The listing builds one solid part. Answer for the finished solid, in the listing's coordinates (mm). Face numbers are marked on the shaded views. A direction names the side the tool comes from. Round coordinates to 2 decimals unless told otherwise and drop trailing zeros. Write each loop counter-clockwise with the first axis right and the second up, starting at its lowest first coordinate (ties: lowest second). Pieces come first, ordered by that corner, then holes.
Item 1: A tool of negligible diameter and unlimited length cuts with its end or side. For the marked faces 4 and 5, from which of +Z, -Z, +X, -X, +Y, -Y can it reach the whole face along a straight path? Write none if from no direction.
Item 2: Find section D-D on y = 26.75. Give the vertices of the cut face in (x, z), then the cut area to 3 significant figures.
Item 3: Find the intervals of material crossed by probe 1 along Z at (x, y) = (0, 23.1); probe 2 along Y at (x, z) = (24.5, -21.5); probe 3 along Z at (x, y) = (2.5, 22.5), in increasing order.
Item 4: Each of these flat-tipped pins is pushed along its axis until it touches: pin 1 (6 mm diameter, centred on y = 25, z = 32, fed in from +X); pin 2 (2.5 mm diameter, centred on x = 0, z = -34.5, fed in from +Y); pin 3 (2.5 mm diameter, centred on x = 0, z = 32.5, fed in from -Y); pin 4 (2 mm diameter, centred on y = 22, z = -21, fed in from -X). Where does it stop, or does it pass through?
Item 5: Find section B-B on x = 17. Give the vertices of the cut face in (y, z), then the cut area to 3 significant figures.
Item 6: Find section A-A on z = -34.5. Give the vertices of the cut face in (x, y), then the cut area to 3 significant figures.
Item 7: Find section C-C on x = 0. Give the number of separate pieces and of enclosed holes in the cut face, then the cut area to 3 significant figures.
Item 8: For a pull along X with two mould halves and no side action, classify the marked faces 1, 2 and 3 as +X half, -X half, draft (parallel to the pull), parting line (faces both ways), or undercut.
Autodesk Inventor part; units mm, degrees
ref_plane "YZ Plane" through (0, 0, 0) normal (1, 0, 0) x (0, 1, 0)
ref_plane "XZ Plane" through (0, 0, 0) normal (0, 1, 0) x (-1, 0, 0)
ref_plane "XY Plane" through (0, 0, 0) normal (0, 0, 1) x (1, 0, 0)
sketch "スケッチ1" plane through (0, 0, 0) normal (0, 1, 0) x (-1, 0, 0)
  circle A0 centre (0, 0) radius 40
  dimension "d0" = 80
extrude "押し出し1" add sketch "スケッチ1" along normal blind 28.6
sketch "スケッチ2" plane through (0, 0, 0) normal (0, -1, 0) x (1, 0, 0)
  circle A0 centre (0, 0) radius 30.05
  circle A1 centre (0, 0) radius 40
  dimension "d3" = 60.1
  dimension "d4" = 80
extrude "押し出し2" cut sketch "スケッチ2" against normal blind 19
sketch "スケッチ3" plane through (0, 0, 0) normal (0, -1, 0) x (1, 0, 0)
  circle A0 centre (0, 0) radius 27.5
  circle A1 centre (0, 0) radius 30.05
  dimension "d7" = 55
extrude "押し出し3" cut sketch "スケッチ3" against normal blind 15
sketch "スケッチ5" plane through (0, 0, 0) normal (0, -1, 0) x (1, 0, 0)
  circle A0 centre (0, 0) radius 20
  dimension "d10" = 40
extrude "押し出し4" cut sketch "スケッチ5" against normal blind 5.5
sketch "スケッチ6" plane through (0, 5.5, 0) normal (0, -1, 0) x (1, 0, 0)
  circle A0 centre (0, 0) radius 6
  dimension "d13" = 12
extrude "押し出し5" cut sketch "スケッチ6" against normal blind 30000
sketch "スケッチ7" plane through (0, 19, 0) normal (0, -1, 0) x (1, 0, 0)
  circle A0 centre (0, 0) radius 34.5
  circle A1 centre (0, 34.5) radius 2
  circle A2 centre (34.5, 0) radius 2
  circle A3 centre (0, -34.5) radius 2
  circle A4 centre (-34.4997, 0.1397) radius 2
  dimension "d60" = 69
  dimension "d61" = 4
  dimension "d62" = 4
  dimension "d63" = 4
  dimension "d64" = 4
extrude "押し出し6" cut sketch "スケッチ7" against normal blind 10 contours A0 A2 | A0 A2 | A1 A0 | A0 A1 | A3 A0 | A0 A3 | A4 A0 | A0 A4
hole "穴1" at (34.5, 19, 0) direction (0, 1, 0) diameter 4.2 depth 10 counterbore diameter 8 counterbore depth 5.4
hole "穴2" at (-34.4997, 19, 0.1397) direction (0, 1, 0) diameter 4.2 depth 10 counterbore diameter 8 counterbore depth 5.4
hole "穴3" at (0, 19, -34.5) direction (0, 1, 0) diameter 4.2 depth 10 counterbore diameter 8 counterbore depth 5.4
hole "穴4" at (0, 19, 34.5) direction (0, 1, 0) diameter 4.2 depth 10 counterbore diameter 8 counterbore depth 5.4
properties part number "GearHead2"
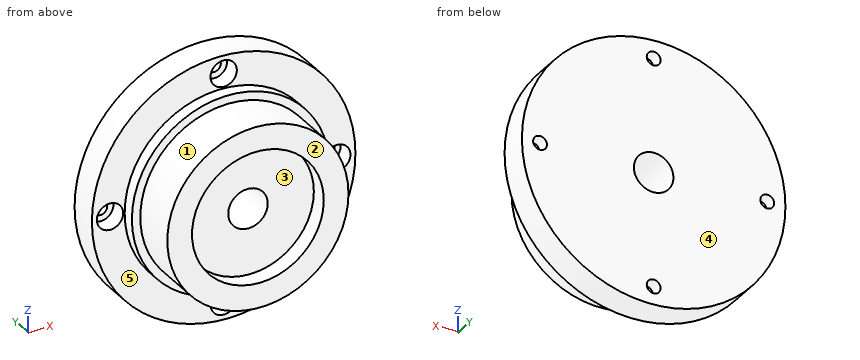
Check values:
1. face 4: +Z, -Z, +X, -X, +Y
1. face 5: -Y
2. outline: circle Ø80 at (0, 0); hole circle Ø4.2 at (-34.5, 0.14); hole circle Ø12 at (0, 0); hole circle Ø4.2 at (0, -34.5); hole circle Ø4.2 at (0, 34.5); hole circle Ø4.2 at (34.5, 0)
2. area: 4,860 mm2
3. probe 1: z = -40 to -38.5, -30.5 to -6, 6 to 30.5, 38.5 to 40
3. probe 2: y = 19 to 28.6
3. probe 3: z = -39.92 to -37.62, -31.38 to -5.45, 5.45 to 31.38, 37.62 to 39.92
4. pin 1: stops at x = 27.55
4. pin 2: passes through
4. pin 3: stops at y = 24.4
4. pin 4: stops at x = -34.64
5. outline: (0, -21.62) - (15, -21.62) - (15, -24.78) - (19, -24.78) - (19, -36.21) - (28.6, -36.21) - (28.6, 36.21) - (19, 36.21) - (19, 24.78) - (15, 24.78) - (15, 21.62) - (0, 21.62) - (0, 10.54) - (5.5, 10.54) - (5.5, -10.54) - (0, -10.54) - close
5. area: 1,430 mm2
6. outline: (-20.24, 19) - (-4, 19) - (-4, 24.4) - (-2.1, 24.4) - (-2.1, 28.6) - (-20.24, 28.6) - close; (2.1, 24.4) - (4, 24.4) - (4, 19) - (20.24, 19) - (20.24, 28.6) - (2.1, 28.6) - close
6. area: 328 mm2
7. separate pieces: 4
7. enclosed holes: 0
7. area: 1,210 mm2
8. face 1: parting line
8. face 2: draft
8. face 3: undercut
